```python
from build123d import *

# Parameters (mm, degrees)
RESSALTO_EXTRUS_O1_DEPTH = 5
ESBO_O2_W                = 6
ESBO_O2_H                = 5
CORTE_EXTRUS_O1_DEPTH    = 10
ESBO_O3_W                = 120
ESBO_O3_H                = 15
RESSALTO_EXTRUS_O2_DEPTH = 5


with BuildPart() as part:
    # Esboço1 → Ressalto-extrusão1 (new body)
    with BuildSketch(Plane(origin=(0, 0, 0), x_dir=(1, 0, 0), z_dir=(0, 1, 0))):
        with BuildLine():
            ThreePointArc((-17.839278071, -21.26900995), (-27.839278071, -11.26900995), (-37.839278071, -21.26900995))
            Line((-37.839278071, -21.26900995), (-17.839278071, -21.26900995))
        make_face()
        with BuildLine():
            Line((-17.839278071, -21.26900995), (-37.839278071, -21.26900995))
            ThreePointArc((-37.839278071, -21.26900995), (-27.839278071, -31.26900995), (-17.839278071, -21.26900995))
        make_face()
        with BuildLine():
            Line((-17.839278071, -5.26900995), (-37.839278071, -5.26900995))
            Line((-37.839278071, -5.26900995), (-37.839278071, -21.26900995))
            ThreePointArc((-37.839278071, -21.26900995), (-27.839278071, -11.26900995), (-17.839278071, -21.26900995))
            Line((-17.839278071, -21.26900995), (-17.839278071, -5.26900995))
        make_face()
    extrude(amount=RESSALTO_EXTRUS_O1_DEPTH)

    # Esboço2 → Corte-extrusão1 (cut)
    with BuildSketch(Plane(origin=(0, 5, 0), x_dir=(1, 0, 0), z_dir=(0, 1, 0))):
        with Locations((-34.839278071, -7.76900995)):
            Rectangle(ESBO_O2_W, ESBO_O2_H)
        with Locations((-20.839278071, -7.76900995)):
            Rectangle(ESBO_O2_W, ESBO_O2_H)
    extrude(amount=-CORTE_EXTRUS_O1_DEPTH, mode=Mode.SUBTRACT)

    # Esboço3 → Ressalto-extrusão2 (add)
    with BuildSketch(Plane(origin=(0, 5, 0), x_dir=(1, 0, 0), z_dir=(0, 1, 0))):
        with Locations((-77.839278071, 2.23099005)):
            Rectangle(ESBO_O3_W, ESBO_O3_H)
    extrude(amount=-RESSALTO_EXTRUS_O2_DEPTH)


solid = part.part
```
Work out the finished part from the listing and answer in its coordinate system (mm). A direction names the side the tool comes from. Give positions to 0.01 mm unless a question says otherwise; leave off trailing zeros. Order: outer loops, then holes, each group sorted by start corner. A loop starts at its lowest first (then second) coordinate and runs counter-clockwise, first axis right, second up. Notation, with made-up numbers: (26, 40) -> (66, 40) arc R6 cw to (66, 50) -> close; hole circle Ø5 at (34, 36.25). An arc over 180 degrees is marked (long way). Answer as CSV lines item,"result". Start each with the question number.
(1) Section B-B, the plane z = 12 is taken. Write down the section's boundary in (x, y), plus the area to 3 significant figures.
(2) For a pull along Z with two mould halves and no side action, classify faces 4 (the flat face through (-17.839, 3, -2)), 5 (the cylindrical face through (-28.059, 2.465, 31.267)), 6 (the flat face through (-21, 3, 5.269)) as released by +Z, released by -Z, zero draft, split by the parting line, or undercut.
(3) Consider line 1 along X through (y, z) = (3.8, 15); line 2 along Z through (x, y) = (-114, 2.65); line 3 along X through (y, z) = (4.25, 7). Determine where each line is inside the solid, lowest interval first.
(4) Each of these flat-tipped pins is pushed along its axis until it touches: pin 1 Ø1.5 at (y, z) = (2.5, 7) entering from -X; pin 2 Ø10 at (x, z) = (-63.5, 11) entering from +Y; pin 3 Ø1.5 at (y, z) = (2, 13) entering from -X. Where does it stop, or does it pass through?
(5) Which of the six approach directions +Z, -Z, +X, -X, +Y, -Y give full straight-line access (tool end or side, diameter ignored) to faces 1 (the flat face through (-21, 3, 10.269)), 2 (the flat face through (-31.839, 3, 8)), 3 (the flat face through (-37.839, 2, 16))?
(6) Section A-A, the plane y = 3.55 is taken. Write down the section's boundary in (x, z), plus the area to 3 significant figures.
(7) Section C-C, the plane x = -79 is taken. Write down the section's boundary in (y, z).
Entries:
1,outline,"(-37.84, 0) -> (-17.84, 0) -> (-17.84, 5) -> (-37.84, 5) -> close"
1,area,"100 mm²"
2,face 4,"zero draft"
2,face 5,"released by +Z"
2,face 6,"undercut"
3,line 1,"-37.84 to -17.84"
3,line 2,"-9.73 to 5.27"
3,line 3,"-31.84 to -23.84"
4,pin 1,"x = -31.84"
4,pin 2,"through"
4,pin 3,"x = -37.84"
5,face 1,"+X, +Y, -Y"
5,face 2,"-X, +Y, -Y"
5,face 3,"+Z, -X, +Y, -Y"
6,outline,"(-137.84, -9.73) -> (-17.84, -9.73) -> (-17.84, 5.27) -> (-23.84, 5.27) -> (-23.84, 10.27) -> (-17.84, 10.27) -> (-17.84, 21.27) arc R10 ccw to (-37.84, 21.27) -> (-37.84, 10.27) -> (-31.84, 10.27) -> (-31.84, 5.27) -> (-137.84, 5.27) -> close"
6,area,"2,220 mm²"
7,outline,"(0, -9.73) -> (5, -9.73) -> (5, 5.27) -> (0, 5.27) -> close"
